Geometry: final body of the model. Coordinates: model frame, mm. Round coordinates to 2 decimals unless told otherwise and drop trailing zeros. Order: outer loops, then holes, each group sorted by start corner. A loop starts at its lowest first (then second) coordinate and runs counter-clockwise, first axis right, second up. Notation, with made-up numbers: M -24.75,-20 L 7.25,-20 A23 ccw 7.25,13 Z; hole C 48.5,-23.5 d10. An arc over 180 degrees is marked long. Return JSON: item names as keys, results as strings. Group by question number.
Q1. Ray query, probe 1 along Y at (x, z) = (-12.5, 1.2); probe 2 along X at (y, z) = (9.25, 4); probe 3 along Y at (x, z) = (15, 0.55). Return the intervals inside material, ascending.
Q2. Mould query, pull axis Y, two halves, no side actions, for faces 1 (the face through (0, 0, 5)), 2 (the face through (-16.07, -12.5, 2.54)), 3 (the face through (-12.63, -8.01, 2.54)), 4 (the face through (16.07, 12.5, 2.54)). Classes: released by +Y, released by -Y, zero draft, split by the parting line, or undercut.
Q3. Contact query for a flat-ended pin moving along its axis: pin 1 (2.5 mm diameter, centred on x = -12.5, y = 9, fed in from +Z). Output: stop coordinate, or through.
Q4. Cut plane B-B on x = -14. Output: boundary loops of the cut face in (y, z), and give its area (3 significant figures).
Q5. Cut plane A-A on z = 4.5. Output: boundary loops of the cut face in (x, y).
```python
from build123d import *

# Parameters (mm, degrees)
SKETCH1_W           = 35
SKETCH1_H           = 28
BOSS_EXTRUDE1_DEPTH = 5
FILLET1_R           = 5
SKETCH2_R           = 1
CUT_EXTRUDE1_DEPTH  = 23.961925006


with BuildPart() as part:
    # Sketch1 → Boss-Extrude1 (new body)
    with BuildSketch(Plane.XY):
        Rectangle(SKETCH1_W, SKETCH1_H)
    extrude(amount=BOSS_EXTRUDE1_DEPTH)

    # Fillet1
    fillet1_edges = [part.edges().sort_by_distance(p)[0] for p in [
        (17.5, 14, 2.5),
        (17.5, -14, 2.5),
        (-17.5, -14, 2.5),
        (-17.5, 14, 2.5),
    ]]
    fillet(fillet1_edges, radius=FILLET1_R)

    # Sketch2 → Cut-Extrude1 (cut, through all)
    with BuildSketch(Plane.XY.offset(5)):
        with Locations((-12.5, -9)):
            Circle(SKETCH2_R)
        with Locations((-12.5, 9)):
            Circle(SKETCH2_R)
        with Locations((12.5, 9)):
            Circle(SKETCH2_R)
        with Locations((12.5, -9)):
            Circle(SKETCH2_R)
    extrude(amount=-CUT_EXTRUDE1_DEPTH, mode=Mode.SUBTRACT)


solid = part.part
```
Result sheet:
{
 "1": {"probe 1": "y = -14 to -10, -8 to 8, 10 to 14", "probe 2": "x = -17.49 to -13.47, -11.53 to 11.53, 13.47 to 17.49", "probe 3": "y = -13.33 to 13.33"},
 "2": {"face 1": "zero draft", "face 2": "released by -Y", "face 3": "undercut", "face 4": "released by +Y"},
 "3": {"pin 1": "stops at z = 5"},
 "4": {"outline": "M -13.77,0 L 13.77,0 L 13.77,5 L -13.77,5 Z", "area": "138 mm²"},
 "5": {"outline": "M -17.5,-9 A5 ccw -12.5,-14 L 12.5,-14 A5 ccw 17.5,-9 L 17.5,9 A5 ccw 12.5,14 L -12.5,14 A5 ccw -17.5,9 Z; hole C -12.5,-9 d2; hole C -12.5,9 d2; hole C 12.5,-9 d2; hole C 12.5,9 d2"}
}
